```python
from build123d import *

# Parameters (mm, degrees)
SWEEP1_PROFILE_R   = 12.7
SKETCH18_R         = 3.175
CUT_EXTRUDE1_DEPTH = 179.704840449
LPATTERN1_COUNT    = 4
LPATTERN1_PITCH    = 25.4
SKETCH19_R         = 3.175
CUT_EXTRUDE2_DEPTH = 179.704840563


with BuildPart() as part:
    # Sweep1: sweep along a path in Sketch1
    with BuildLine(Plane.XY) as sweep1_path:
        Line((0, 0), (177.8, 0))
    # Sweep1 profile (on start of the path) → Sweep1 (sweep)
    with BuildSketch(Plane(origin=(0, 0, 0), x_dir=(0, 0, 1), z_dir=(1, 0, 0))):
        Circle(SWEEP1_PROFILE_R)
    sweep(path=sweep1_path.line)

    # Sketch18 → Cut-Extrude1 (cut, through all)
    with BuildSketch(Plane.XY):
        with Locations((139.7, 0)):
            Circle(SKETCH18_R)
    cut_extrude1 = extrude(amount=-CUT_EXTRUDE1_DEPTH, mode=Mode.SUBTRACT)

    # LPattern1: Cut-Extrude1 ×4
    with Locations(*[(-i * LPATTERN1_PITCH, 0, 0) for i in range(1, LPATTERN1_COUNT)]):
        add(cut_extrude1, mode=Mode.SUBTRACT)

    # Sketch19 → Cut-Extrude2 (cut, through all)
    with BuildSketch(Plane(origin=(0, 0, 0), x_dir=(-1, 0, 0), z_dir=(0, 0, -1))):
        with Locations((-63.5, 0)):
            Circle(SKETCH19_R)
    extrude(amount=-CUT_EXTRUDE2_DEPTH, mode=Mode.SUBTRACT)


solid = part.part
```
Read the model definition and answer for the solid it produces. Units are mm, in the model's axes. Give positions to 0.01 mm unless a question says otherwise; leave off trailing zeros. Write each loop counter-clockwise with the first axis right and the second up, starting at its lowest first coordinate (ties: lowest second). Pieces come first, ordered by that corner, then holes. Notation, with made-up numbers: M 21,73 L 44,73 A20 ccw 44,102 Z; hole C 70.25,-5.75 d7. An arc over 180 degrees is marked long. Put each result on its own line as item: value. Start each with the question number.
1. The part is cut by section B-B, the plane z = -4.75. Give the vertices of the cut face in (x, y) (3 decimals).
2. The part is cut by section C-C, the plane x = 63.5. Give the vertices of the cut face in (y, z) (3 decimals), and give its area (3 significant figures).
3. Each of these flat-tipped pins is pushed along its axis until it touches: pin 1 Ø1.9 at (x, y) = (90.5, -1) entering from -Z; pin 2 Ø10 at (x, y) = (115.5, 8) entering from -Z; pin 3 Ø8 at (x, z) = (61, 4.5) entering from -Y. Where does it stop, or does it pass through?
4. Consider line 1 along X through (y, z) = (0, -7) (3 decimals); line 2 along Z through (x, y) = (162, -0.5); line 3 along Y through (x, z) = (139.7, -9.5) (3 decimals). Determine where each line is inside the solid, lowest interval first.
5. The part is cut by section D-D, the plane x = 151. Give the vertices of the cut face in (y, z), and give its area (3 significant figures).
6. For a pull along X with two mould halves and no side action, classify faces 1 (the flat face through (177.8, 0, 0)), 2 (the cylindrical face through (90.145, -3.815, 12.114)), 3 (the flat face through (89, 0, 0)), 4 (the flat face through (0, 0, 0)) as released by +X, released by -X, zero draft, split by the parting line, or undercut.
7. The part is cut by section A-A, the plane y = 0. Give the vertices of the cut face in (x, z) (3 decimals), and give its area (3 significant figures).
Final values:
1. outline: M 0,-11.778 L 177.8,-11.778 L 177.8,11.778 L 0,11.778 Z; hole C 63.5,0 d6.35; hole C 88.9,0 d6.35; hole C 114.3,0 d6.35; hole C 139.7,0 d6.35
2. outline: M -3.175,-12.297 L -3.175,12.297 A12.7 ccw Z; M 3.175,-12.297 A12.7 ccw 3.175,12.297 Z
2. area: 347 mm²
3. pin 1: stops at z = 0
3. pin 2: stops at z = -12.34
3. pin 3: stops at y = -12.69
4. line 1: x = 0 to 60.325, 66.675 to 85.725, 92.075 to 111.125, 117.475 to 136.525, 142.875 to 177.8
4. line 2: z = -12.69 to 12.69
4. line 3: y = -8.429 to -3.175, 3.175 to 8.429
5. outline: C 0,0 d25.4
5. area: 507 mm²
6. face 1: released by +X
6. face 2: zero draft
6. face 3: undercut
6. face 4: released by -X
7. outline: M 0,-12.7 L 60.325,-12.7 L 60.325,12.7 L 0,12.7 Z; M 66.675,-12.7 L 85.725,-12.7 L 85.725,0 L 92.075,0 L 92.075,-12.7 L 111.125,-12.7 L 111.125,0 L 117.475,0 L 117.475,-12.7 L 136.525,-12.7 L 136.525,0 L 142.875,0 L 142.875,-12.7 L 177.8,-12.7 L 177.8,12.7 L 66.675,12.7 Z
7. area: 4,110 mm²
